For this review, take the finished solid that the model builds, in its own axes (mm). A direction names the side the tool comes from. Give positions to 0.01 mm unless a question says otherwise; leave off trailing zeros. Order: outer loops, then holes, each group sorted by start corner. A loop starts at its lowest first (then second) coordinate and runs counter-clockwise, first axis right, second up. Notation, with made-up numbers: (77, 25.5) - (120, 25.5) arc R34 ccw to (120, 56.5) - close; hole circle Ø5 at (-20, 11). An arc over 180 degrees is marked (long way). One line per item, written item: value.
```python
from build123d import *

# Parameters (mm, degrees)
SKETCH1_W              = 45
SKETCH1_H              = 20
BOSS_EXTRUDE2_DEPTH    = 1.5
SKETCH2_R              = 8
SKETCH2_R_2            = 7.072496476
BOSS_EXTRUDE3_DEPTH    = 12
BOSS_EXTRUDE4_DEPTH    = 2
SKETCH4_R              = 0.730672048
CUT_EXTRUDE6_DEPTH     = 22
SKETCH7_R              = 0.66039865
CUT_EXTRUDE9_DEPTH     = 11
SKETCH9_W              = 2
SKETCH9_H              = 2
BOSS_EXTRUDE5_DEPTH    = 2
FILLET2_R              = 0.2
LPATTERN1_COUNT        = 4
LPATTERN1_PITCH        = 2.1
FILLET2_OF_LPATTERN1_R = 0.2


with BuildPart() as part:
    # Sketch1 → Boss-Extrude2 (new body)
    with BuildSketch(Plane(origin=(0, 0, 0), x_dir=(1, 0, 0), z_dir=(0, 1, 0))):
        with Locations((-31.512400592, -30.621028873)):
            Rectangle(SKETCH1_W, SKETCH1_H)
    extrude(amount=BOSS_EXTRUDE2_DEPTH)

    # Sketch2 → Boss-Extrude3 (add)
    # profile 1 of 2: a face of its own
    with BuildSketch(Plane(origin=(0, 1.5, 0), x_dir=(1, 0, 0), z_dir=(0, 1, 0))):
        with Locations(Location((-44.251420367, -30.391308844, 0), (0, 0, 90))):
            Circle(SKETCH2_R)
        with Locations(Location((-44.251420367, -30.391308844, 0), (0, 0, 270))):
            Circle(SKETCH2_R_2, mode=Mode.SUBTRACT)
    # profile 2 of 2: a face of its own
    with BuildSketch(Plane(origin=(0, 1.5, 0), x_dir=(1, 0, 0), z_dir=(0, 1, 0))):
        with Locations(Location((-18.773380818, -30.391308844, 0), (0, 0, 90))):
            Circle(SKETCH2_R)
        with Locations(Location((-18.773380818, -30.391308844, 0), (0, 0, 90))):
            Circle(SKETCH2_R_2, mode=Mode.SUBTRACT)
    extrude(amount=BOSS_EXTRUDE3_DEPTH)

    # Sketch3 → Boss-Extrude4 (add)
    with BuildSketch(Plane(origin=(0, 1.5, 0), x_dir=(1, 0, 0), z_dir=(0, 1, 0))):
        with BuildLine():
            Line((-35.62647747, -21.369576807), (-27.62647747, -21.369576807))
            ThreePointArc((-27.62647747, -21.369576807), (-26.081088186, -22.914966091), (-27.62647747, -24.460355375))
            Line((-27.62647747, -24.460355375), (-35.62647747, -24.460355375))
            ThreePointArc((-35.62647747, -24.460355375), (-37.171866754, -22.914966091), (-35.62647747, -21.369576807))
        make_face()
    extrude(amount=BOSS_EXTRUDE4_DEPTH)

    # Sketch4 → Cut-Extrude6 (cut)
    with BuildSketch(Plane(origin=(0, 1.5, 0), x_dir=(1, 0, 0), z_dir=(0, 1, 0))):
        with Locations(Location((-51.851239407, -38.465008216, 0), (0, 0, 270))):
            Circle(SKETCH4_R)
    extrude(amount=-CUT_EXTRUDE6_DEPTH, mode=Mode.SUBTRACT)

    # Sketch7 → Cut-Extrude9 (cut)
    with BuildSketch(Plane(origin=(0, 1.5, 0), x_dir=(1, 0, 0), z_dir=(0, 1, 0))):
        with Locations(Location((-10.921132564, -22.246689644, 0), (0, 0, 270))):
            Circle(SKETCH7_R)
    extrude(amount=-CUT_EXTRUDE9_DEPTH, mode=Mode.SUBTRACT)

    # Sketch9 → Boss-Extrude5 (add)
    with BuildSketch(Plane.XZ):
        with Locations((-28.362400592, 38.253484629)):
            Rectangle(SKETCH9_W, SKETCH9_H)
    boss_extrude5 = extrude(amount=BOSS_EXTRUDE5_DEPTH)

    # Fillet2
    fillet2_edges = [part.edges().sort_by_distance(p)[0] for p in [
        (-27.362400592, -1, 37.253484629),
        (-27.362400592, -1, 39.253484629),
        (-29.362400592, -1, 39.253484629),
        (-29.362400592, -1, 37.253484629),
    ]]
    fillet(fillet2_edges, radius=FILLET2_R)

    # LPattern1: Boss-Extrude5 ×4
    with Locations(*[(-i * LPATTERN1_PITCH, 0, 0) for i in range(1, LPATTERN1_COUNT)]):
        add(boss_extrude5)

    # Fillet2 of LPattern1
    fillet2_of_lpattern1_edges = [part.edges().sort_by_distance(p)[0] for p in [
        (-29.462400592, -1, 37.253484629),
        (-29.462400592, -1, 39.253484629),
        (-31.462400592, -1, 39.253484629),
        (-31.462400592, -1, 37.253484629),
        (-31.562400592, -1, 37.253484629),
        (-31.562400592, -1, 39.253484629),
        (-33.562400592, -1, 39.253484629),
        (-33.562400592, -1, 37.253484629),
        (-33.662400592, -1, 37.253484629),
        (-33.662400592, -1, 39.253484629),
        (-35.662400592, -1, 39.253484629),
        (-35.662400592, -1, 37.253484629),
    ]]
    fillet(fillet2_of_lpattern1_edges, radius=FILLET2_OF_LPATTERN1_R)


solid = part.part
```
(1) Take a section at D-D (x = -30.5). Write out the cut boundary in (y, z), then the cut area to 3 significant figures.
Answers below:
outline: (-2, 37.25) - (0, 37.25) - (0, 20.62) - (1.5, 20.62) - (1.5, 21.37) - (3.5, 21.37) - (3.5, 24.46) - (1.5, 24.46) - (1.5, 40.62) - (0, 40.62) - (0, 39.25) - (-2, 39.25) - close
area: 40.2 mm^2
(2) Machinability: for faces 4 (the face through (-33, -1, 37.253)), 5 (the face through (-32, 2, 21.37)), 6 (the face through (-35.662, -1, 38)), 7 (the face through (-43.94, 7.416, 23.326)), which of the approach directions +Z, -Z, +X, -X, +Y, -Y give a long, thin tool a straight path to every point of the face, cutting with its end or side? Answer none if there is none.
Answers below:
face 4: -Z, +X, -X, -Y
face 5: -Z, +X, -X, +Y
face 6: +Z, -Z, -X, -Y
face 7: +Y
(3) Take a section at A-A (y = -1). Give the number of separate pieces and of enclosed holes in the cut face, then the cut area to 3 significant figures.
Answers below:
separate pieces: 4
enclosed holes: 0
area: 15.9 mm^2
(4) Draft analysis for pull direction Z (two halves, no side actions). For faces 1 (the face through (-13, 13.5, 26)), 2 (the face through (-26.08, 2.49, 22.88)), 3 (the face through (-30, -1, 39.253)), state which applies: pulls with the +Z half, pulls with the -Z half, needs draft (parallel to the pull), parting line crosses it, or undercut.
Answers below:
face 1: needs draft
face 2: undercut
face 3: pulls with the +Z half
(5) Take a section at C-C (z = 35.5). Write out the cut boundary in (x, y).
Answers below:
outline: (-54.01, 0) - (-9.01, 0) - (-9.01, 1.5) - (-12.62, 1.5) - (-12.62, 13.5) - (-13.88, 13.5) - (-13.88, 1.5) - (-23.66, 1.5) - (-23.66, 13.5) - (-24.93, 13.5) - (-24.93, 1.5) - (-38.1, 1.5) - (-38.1, 13.5) - (-39.36, 13.5) - (-39.36, 1.5) - (-49.14, 1.5) - (-49.14, 13.5) - (-50.41, 13.5) - (-50.41, 1.5) - (-54.01, 1.5) - close
(6) Wall thickness on line 1 (X direction, y = 11.75, z = 30.25); line 2 (X direction, y = 7.5, z = 34.75); line 3 (Y direction, x = -30.5, z = 26): over which ranges is each line inside the solid? List them lowest first. Write a range as from..to.
Answers below:
line 1: x = -52.25..-51.32, -37.18..-36.25, -26.77..-25.84, -11.7..-10.77
line 2: x = -50.96..-49.82, -38.68..-37.54, -25.48..-24.34, -13.2..-12.07
line 3: y = 0..1.5
(7) For P1, Ø2, axis at y = 9, z = 29.5, coming from the -X side; P2, Ø4, axis at x = -46, z = 30, coming from the +Y side; P3, Ø12, axis at x = -40, z = 34.5, coming from the +Y side; P4, Ø10, axis at x = -25, z = 31, coming from the -Y side, all flat-tipped, find the tip position at first contact; note any pin that passes through.
Answers below:
P1: stops at x = -52.25
P2: stops at y = 1.5
P3: stops at y = 13.5
P4: stops at y = 0
(8) Take a section at B-B (y = 3). Write out the cut boundary in (x, z) (1 decimal).
Answers below:
outline: circle Ø16 at (-44.3, 30.4); (-35.6, 21.4) - (-27.6, 21.4) arc R1.5 ccw to (-27.6, 24.5) - (-35.6, 24.5) arc R1.5 ccw to start; circle Ø16 at (-18.8, 30.4); hole circle Ø14.1 at (-44.3, 30.4); hole circle Ø14.1 at (-18.8, 30.4)
